Design review of the part built by this model. Coordinates are the model's own, in mm. A direction names the side the tool comes from. Round coordinates to 2 decimals unless told otherwise and drop trailing zeros. Write each loop counter-clockwise with the first axis right and the second up, starting at its lowest first coordinate (ties: lowest second). Pieces come first, ordered by that corner, then holes. Notation, with made-up numbers: (44.5, 35.5) - (73.5, 35.5) arc R30 cw to (73.5, 68.5) - close; hole circle Ø9 at (23.5, 76.25). An arc over 180 degrees is marked (long way). Use one line per item in the form item = value.
```python
from build123d import *

# Parameters (mm, degrees)
SKETCH3_W           = 52
SKETCH3_H           = 52
BOSS_EXTRUDE1_DEPTH = 40
SKETCH4_R           = 3
CUT_EXTRUDE5_DEPTH  = 40
SKETCH4_5_R         = 9.5
SKETCH4_5_R_2       = 3
CUT_EXTRUDE6_DEPTH  = 6
CUT_EXTRUDE8_START  = -6
SKETCH5_R           = 9.5
CUT_EXTRUDE8_DEPTH  = 6
SKETCH6_W           = 10
SKETCH6_H           = 52
BOSS_EXTRUDE2_DEPTH = 5
SKETCH7_R           = 2
CUT_EXTRUDE9_DEPTH  = 5


with BuildPart() as part:
    # Sketch3 → Boss-Extrude1 (new body)
    with BuildSketch(Plane.XY):
        Rectangle(SKETCH3_W, SKETCH3_H)
    extrude(amount=BOSS_EXTRUDE1_DEPTH)

    # Sketch4 → Cut-Extrude5 (cut)
    with BuildSketch(Plane.XY.offset(40)):
        Circle(SKETCH4_R)
    extrude(amount=-CUT_EXTRUDE5_DEPTH, mode=Mode.SUBTRACT)

    # Sketch4<5> → Cut-Extrude6 (cut)
    with BuildSketch(Plane.XY.offset(40)):
        Circle(SKETCH4_5_R)
        Circle(SKETCH4_5_R_2, mode=Mode.SUBTRACT)
    extrude(amount=-CUT_EXTRUDE6_DEPTH, mode=Mode.SUBTRACT)

    # Sketch5 → Cut-Extrude8 (cut)
    with BuildSketch(Plane(origin=(0, 0, 0), x_dir=(-1, 0, 0), z_dir=(0, 0, -1)).offset(CUT_EXTRUDE8_START)):
        with Locations(Location((0, 0, 0), (0, 0, 180))):
            Circle(SKETCH5_R)
    extrude(amount=CUT_EXTRUDE8_DEPTH, mode=Mode.SUBTRACT)

    # Sketch6 → Boss-Extrude2 (add)
    with BuildSketch(Plane.XY.offset(40)):
        with Locations((31, 0)):
            Rectangle(SKETCH6_W, SKETCH6_H)
        with Locations((-31, 0)):
            Rectangle(SKETCH6_W, SKETCH6_H)
    extrude(amount=-BOSS_EXTRUDE2_DEPTH)

    # Sketch7 → Cut-Extrude9 (cut)
    with BuildSketch(Plane(origin=(0, 0, 35), x_dir=(-1, 0, 0), z_dir=(0, 0, -1))):
        with Locations((-32, 17.5)):
            Circle(SKETCH7_R)
        with Locations((32, 17.5)):
            Circle(SKETCH7_R)
        with Locations((32, -17.5)):
            Circle(SKETCH7_R)
        with Locations((-32, -17.5)):
            Circle(SKETCH7_R)
    extrude(amount=-CUT_EXTRUDE9_DEPTH, mode=Mode.SUBTRACT)


solid = part.part
```
Q1. We need section C-C on y = 0. Write out the cut boundary in (x, z).
Calculated:
outline = (-36, 35) - (-26, 35) - (-26, 0) - (-9.5, 0) - (-9.5, 6) - (-3, 6) - (-3, 34) - (-9.5, 34) - (-9.5, 40) - (-36, 40) - close; (3, 6) - (9.5, 6) - (9.5, 0) - (26, 0) - (26, 35) - (36, 35) - (36, 40) - (9.5, 40) - (9.5, 34) - (3, 34) - close
Q2. For P1, Ø1, axis at y = -11, z = 4.5, coming from the +X side; P2, Ø10.5, axis at y = -4.5, z = 18.5, coming from the -X side; P3, Ø11, axis at x = 33.5, y = 12, coming from the -Z side; P4, Ø24.5, axis at x = 0, y = 0, coming from the -Z side, all flat-tipped, find the tip position at first contact; note any pin that passes through.
Calculated:
P1 = 26
P2 = -26
P3 = 35
P4 = 0
Q3. Machinability: for faces 1 (the flat face through (-9, 6, 40)), 2 (the flat face through (31, 0, 35)), 3 (the flat face through (-26, 0, 17)), 4 (the flat face through (-2.24, -2.24, 6)), 5 (the flat face through (-2.24, 2.24, 34)), which of the approach directions +Z, -Z, +X, -X, +Y, -Y give a long, thin tool a straight path to every point of the face, cutting with its end or side? Answer none if there is none.
Calculated:
face_1 = +Z, +X, -X, +Y, -Y
face_2 = -Z, +X, +Y, -Y
face_3 = -Z, -X, +Y, -Y
face_4 = -Z
face_5 = +Z
Q4. Draft analysis for pull direction Y (two halves, no side actions). For faces 6 (the flat face through (-1, 26, 20)), 7 (the flat face through (26, 0, 17)), 8 (the cylindrical face through (4.38, -8.43, 37.04)), state which applies: released by +Y, released by -Y, zero draft, split by the parting line, or undercut.
Calculated:
face_6 = released by +Y
face_7 = zero draft
face_8 = undercut
Q5. To check wall thickness, follow line 1 along Y through (x, z) = (32, 39.05); line 2 along Y through (x, z) = (0, 37); line 3 along X through (y, z) = (-21.5, 3.5). State the ranges of each line that lie inside material, in increasing order. Write a range as from..to.
Calculated:
line_1 = -26..-19.5, -15.5..15.5, 19.5..26
line_2 = -26..-9.5, 9.5..26
line_3 = -26..26
Q6. We need section B-B on x = -32. Write out the cut boundary in (y, z), then the cut area to 3 significant figures.
Calculated:
outline = (-26, 35) - (-19.5, 35) - (-19.5, 40) - (-26, 40) - close; (-15.5, 35) - (15.5, 35) - (15.5, 40) - (-15.5, 40) - close; (19.5, 35) - (26, 35) - (26, 40) - (19.5, 40) - close
area = 220 mm2
Q7. We need section A-A on y = 17.5. Write out the cut boundary in (x, z).
Calculated:
outline = (-36, 35) - (-34, 35) - (-34, 40) - (-36, 40) - close; (-30, 35) - (-26, 35) - (-26, 0) - (26, 0) - (26, 35) - (30, 35) - (30, 40) - (-30, 40) - close; (34, 35) - (36, 35) - (36, 40) - (34, 40) - close
Q8. We need section D-D on z = 4.5. Write out the cut boundary in (x, y).
Calculated:
outline = (-26, -26) - (26, -26) - (26, 26) - (-26, 26) - close; hole circle Ø19 at (0, 0)
